```python
from build123d import *

# Parameters (mm, degrees)
BOSS_EXTRUDE1_DEPTH     = 15.295
CUT_EXTRUDE1_DEPTH      = 206.919868261
FLOOR_START             = 3
FLOOR_2_DEPTH           = 3
BOSS_EXTRUDE4_START     = 9.785
BOSS_EXTRUDE4_DEPTH     = 9.785
CUT_EXTRUDE3_REACH      = 207.92
CUT_EXTRUDE3_END_RADIUS = 20.596434206
SKETCH7_R               = 5.25
BOSS_EXTRUDE5_REACH     = 176.665
SKETCH14_OUTSIDE_W      = 59.009
SKETCH14_OUTSIDE_H      = 36.805
CUT_EXTRUDE4_DEPTH      = 33.295


with BuildPart() as part:
    # Sketch1 → Boss-Extrude1 (new body)
    with BuildSketch(Plane(origin=(0, 0, -12.295), x_dir=(-1, 0, 0), z_dir=(0, 0, -1))):
        with BuildLine():
            Line((-169.369133898, -111.490025098), (-130.678433581, -111.48937301))
            ThreePointArc((-130.678433581, -111.48937301), (-127.534095849, -100.145401406), (-130.522109497, -88.759255177))
            Line((-130.522109497, -88.759255177), (-169.350721063, -88.778648203))
            ThreePointArc((-169.350721063, -88.778648203), (-172.450070697, -100.131831373), (-169.369133898, -111.490025098))
        make_face()
    extrude(amount=-BOSS_EXTRUDE1_DEPTH)

    # Sketch2 → Cut-Extrude1 (cut, through all)
    with BuildSketch(Plane.XY.offset(3)):
        with BuildLine():
            Line((168.171133654, -90.778059306), (131.717568579, -90.759852501))
            ThreePointArc((131.717568579, -90.759852501), (129.534116109, -100.141151153), (131.855022492, -109.48939284))
            Line((131.855022492, -109.48939284), (168.187605365, -109.490005184))
            ThreePointArc((168.187605365, -109.490005184), (170.450070154, -100.132033398), (168.171133654, -90.778059306))
        make_face()
    extrude(amount=-CUT_EXTRUDE1_DEPTH, mode=Mode.SUBTRACT)

    # Sketch4 → floor 2 (add)
    with BuildSketch(Plane(origin=(0, 0, -12.295), x_dir=(-1, 0, 0), z_dir=(0, 0, -1)).offset(FLOOR_START)):
        with BuildLine():
            Line((-169.369133898, -111.490025098), (-130.678433581, -111.48937301))
            ThreePointArc((-130.678433581, -111.48937301), (-127.534095849, -100.145401406), (-130.522109497, -88.759255177))
            Line((-130.522109497, -88.759255177), (-169.350721063, -88.778648203))
            ThreePointArc((-169.350721063, -88.778648203), (-172.450070697, -100.131831373), (-169.369133898, -111.490025098))
        make_face()
    extrude(amount=-FLOOR_2_DEPTH)

    # Sketch6 → Boss-Extrude4 (add)
    with BuildSketch(Plane.XY.offset(-12.295).offset(BOSS_EXTRUDE4_START)):
        with BuildLine():
            Line((146.5, -90.767235615), (146.5, -108.989639664))
            Line((146.5, -108.989639664), (168.187605365, -109.490005184))
            ThreePointArc((168.187605365, -109.490005184), (170.450070154, -100.132033398), (168.171133654, -90.778059306))
            Line((168.171133654, -90.778059306), (146.5, -90.767235615))
        make_face()
    extrude(amount=-BOSS_EXTRUDE4_DEPTH)

    # Cut-Extrude3: up to this cylinder (the profile starts outside it)
    cut_extrude3_end = Plane(origin=(150.129995683, -99.990000393, -7.995), z_dir=(0, 0, 1)) * Cylinder(CUT_EXTRUDE3_END_RADIUS, 458.032868411, mode=Mode.PRIVATE)
    # Sketch7 → Cut-Extrude3 (cut, up to the surface)
    with BuildSketch(Plane(origin=(0, 0, 0), x_dir=(0, 0, -1), z_dir=(1, 0, 0)), mode=Mode.PRIVATE) as cut_extrude3_sk1:
        with Locations(Location((7.995, -100, 0), (0, 0, 180))):
            Circle(SKETCH7_R)
    cut_extrude3_tool1 = extrude(cut_extrude3_sk1.sketch, amount=CUT_EXTRUDE3_REACH, mode=Mode.PRIVATE) - cut_extrude3_end
    add(cut_extrude3_tool1.solids().sort_by_distance((0, -100, -7.995))[0], mode=Mode.SUBTRACT)

    # Boss-Extrude5: up to this face of the body (flat: up to its plane)
    boss_extrude5_end = Plane(part.part.faces().sort_by_distance((150.023783739, -111.489699054, -6.1475))[0])
    # Sketch11 → Boss-Extrude5 (add, up to the picked face)
    with BuildSketch(Plane(origin=(-0.044298414, -88.694043528, 0), x_dir=(0.9999998752738909, -0.0004994519023308322, 0), z_dir=(0.0004994519023308322, 0.9999998752738909, 0)), mode=Mode.PRIVATE) as boss_extrude5_sk1:
        Polygon((150.03815576, 15.295), (166.500079456, 30.295), (172.500079456, 30.295), (172.500079456, 15.295), align=None)
    boss_extrude5_tool1 = split(extrude(boss_extrude5_sk1.sketch, amount=-BOSS_EXTRUDE5_REACH, mode=Mode.PRIVATE), bisect_by=boss_extrude5_end, keep=Keep.BOTH, mode=Mode.PRIVATE)
    boss_extrude5 = boss_extrude5_tool1.solids().sort_by(Axis((164.546837, -88.776249, -21.34904), (-0.0004994519023308322, -0.9999998752738909, 0)))[0]
    add(boss_extrude5)

    # Mirror1: Boss-Extrude5 across plane
    add(boss_extrude5.mirror(Plane(origin=(149.98984246, -0.002527909, 0), x_dir=(0, 0, 1), z_dir=(-0.9999999998579736, 1.6853871084051315e-05, 0))))

    # Sketch14 outside → Cut-Extrude4 (cut)
    with BuildSketch(Plane.XY.offset(3)):
        with Locations((149.9885, -100.1245)):
            Rectangle(SKETCH14_OUTSIDE_W, SKETCH14_OUTSIDE_H)
        with BuildLine():
            Line((169.350721063, -88.778648203), (130.522109497, -88.759255177))
            ThreePointArc((130.522109497, -88.759255177), (127.534095849, -100.145401406), (130.678433581, -111.48937301))
            Line((130.678433581, -111.48937301), (169.369133898, -111.490025098))
            ThreePointArc((169.369133898, -111.490025098), (172.450070697, -100.131831373), (169.350721063, -88.778648203))
        make_face(mode=Mode.SUBTRACT)
    extrude(amount=-CUT_EXTRUDE4_DEPTH, mode=Mode.SUBTRACT)


solid = part.part
```
CAD build for the part. Positions are in the model's coordinates, mm. A direction names the side the tool comes from. Round coordinates to 2 decimals unless told otherwise and drop trailing zeros. Order: outer loops, then holes, each group sorted by start corner. A loop starts at its lowest first (then second) coordinate and runs counter-clockwise, first axis right, second up.
Item 1: Probe line 1 along Y through (x, z) = (145, -8.5); line 2 along Z through (x, y) = (129.1, -100) (3 decimals); line 3 along Y through (x, z) = (139.5, -23). List the from-to ranges inside material, lowest first.
Item 2: Saw through at D-D on y = -91.75. Write the cut outline in (x, z) (3 decimals).
Item 3: Pin check, flat tips, straight feed: pin 1 (5 mm diameter, centred on x = 133.5, z = -24.5, fed in from +Y); pin 2 (12 mm diameter, centred on x = 150, y = -91.5, fed in from -Z); pin 3 (1.5 mm diameter, centred on y = -108.5, z = -16, fed in from +X). Stop position of each tip, or through.
Item 4: Saw through at B-B on z = -26. Write the cut outline in (x, y).
Item 5: Saw through at A-A on y = -102.5. Write the cut outline in (x, z) (3 decimals), then the cut area to 3 significant figures.
Item 6: Mould opens along X. For faces 1 (the face through (131, -100, -30.295)), 2 (the face through (129.534, -99.958, -12.664)), 3 (the face through (141, -100, -12.295)), 4 (the face through (172.45, -99.97, -13.88)) say: pulls with the +X half, pulls with the -X half, needs draft (parallel to the pull), parting line crosses it, or undercut.
Item 7: Tool access for faces 5 (the face through (146.5, -100, -7)), 6 (the face through (127.534, -99.979, -13.414)), 7 (the face through (128.855, -94.875, -9.133)): list every direction of +Z, -Z, +X, -X, +Y, -Y with a clear straight run to the whole face (end or side of a thin tool).
Reported:
1. line 1: y = -111.49 to -109.49, -90.77 to -88.77
1. line 2: z = -30.295 to -13.245, -2.745 to 3
1. line 3: y = -111.49 to -88.77
2. outline: (129.09, -30.295) - (133.522, -30.295) - (149.984, -15.295) - (149.992, -15.295) - (166.454, -30.295) - (170.816, -30.295) - (170.816, 3) - (168.641, 3) - (168.641, -2.51) - (146.5, -2.51) - (146.5, -12.295) - (131.254, -12.295) - (131.254, 3) - (129.09, 3) - close
3. pin 1: stops at y = -88.78
3. pin 2: stops at z = -20.77
3. pin 3: stops at x = 171.12
4. outline: (130.51, -88.78) arc R22.6 ccw to (130.68, -111.49) - (138.25, -111.49) - (138.23, -88.77) - close; (161.73, -111.49) - (169.37, -111.49) arc R22.41 ccw to (169.35, -88.78) - (161.74, -88.77) - close
5. outline: (127.673, -30.295) - (133.527, -30.295) - (149.988, -15.296) - (166.449, -30.295) - (172.327, -30.295) - (172.327, 3) - (170.314, 3) - (170.314, -2.51) - (146.5, -2.51) - (146.5, -12.295) - (129.687, -12.295) - (129.687, -12.612) - (127.673, -12.612) - close; (127.673, -3.378) - (129.687, -3.378) - (129.687, 3) - (127.673, 3) - close
5. area: 833 mm2
6. face 1: needs draft
6. face 2: pulls with the -X half
6. face 3: undercut
6. face 4: pulls with the +X half
7. face 5: +Z
7. face 6: +Z, -Z, -X
7. face 7: -X
